Geometry check sheet. Reference: the model listing, model coordinates, mm. A direction names the side the tool comes from. Round coordinates to 2 decimals unless told otherwise and drop trailing zeros. Order: outer loops, then holes, each group sorted by start corner. A loop starts at its lowest first (then second) coordinate and runs counter-clockwise, first axis right, second up. Notation, with made-up numbers: (27.25, 81) - (74.25, 81) arc R38 ccw to (74.25, 119) - close; hole circle Ø1 at (25.25, -9). An arc over 180 degrees is marked (long way). Write each question's results on one line, items separated by ' | '.
```python
from build123d import *

# Parameters (mm, degrees)
SKETCH041_W     = 14
SKETCH041_H     = 48
PAD017_DEPTH    = 2
SKETCH043_W     = 10.7
SKETCH043_H     = 16.95
SKETCH043_H_2   = 5
PAD018_DEPTH    = 2
SKETCH044_W     = 10.7
SKETCH044_H     = 2
PAD019_DEPTH    = 11
SKETCH045_R     = 1.6
POCKET019_DEPTH = 5
CHAMFER002_SIZE = 1.5
FILLET006_R     = 1.5
FILLET007_R     = 1
FILLET008_R     = 1


with BuildPart() as part:
    # Sketch041 → Pad017 (new body)
    with BuildSketch(Plane.XY):
        with Locations((-17, -34)):
            Rectangle(SKETCH041_W, SKETCH041_H)
    extrude(amount=PAD017_DEPTH)

    # Sketch043 (on Face5 of Pad017) → Pad018 (join)
    with BuildSketch(Plane(origin=(0, 0, 0), x_dir=(1, 0, 0), z_dir=(0, 0, -1))):
        with Locations((-17, 26.525)):
            Rectangle(SKETCH043_W, SKETCH043_H)
        with Locations((-17, 53.45)):
            Rectangle(SKETCH043_W, SKETCH043_H_2)
    extrude(amount=PAD018_DEPTH)

    # Sketch044 (on Face4 of Pad018) → Pad019 (join)
    with BuildSketch(Plane(origin=(0, 0, 0), x_dir=(1, 0, 0), z_dir=(0, 0, -1))):
        with Locations((-17, 11)):
            Rectangle(SKETCH044_W, SKETCH044_H)
    extrude(amount=PAD019_DEPTH)

    # Sketch045 (on Face5 of Pad019) → Pocket019 (cut)
    with BuildSketch(Plane.XY.offset(2)):
        with Locations((-14.5, -30)):
            Circle(SKETCH045_R)
        with Locations((-17, -54.25)):
            Circle(SKETCH045_R)
    extrude(amount=-POCKET019_DEPTH, mode=Mode.SUBTRACT)

    # Chamfer002
    chamfer002_edges = [part.edges().sort_by_distance(p)[0] for p in [
        (-16.1, -30, 2),
        (-18.6, -54.25, 2),
    ]]
    chamfer(chamfer002_edges, length=CHAMFER002_SIZE)

    # Fillet006
    fillet006_edges = [part.edges().sort_by_distance(p)[0] for p in [
        (-10, -58, 1),
        (-24, -58, 1),
        (-24, -10, 1),
        (-10, -10, 1),
    ]]
    fillet(fillet006_edges, radius=FILLET006_R)

    # Fillet007
    fillet007_edges = [part.edges().sort_by_distance(p)[0] for p in [
        (-24, -34, 2),
    ]]
    fillet(fillet007_edges, radius=FILLET007_R)

    # Fillet008
    fillet008_edges = [part.edges().sort_by_distance(p)[0] for p in [
        (-22.35, -55.95, -1),
        (-11.65, -55.95, -1),
        (-22.35, -35, -1),
        (-11.65, -35, -1),
        (-11.65, -12, -5.5),
        (-22.35, -12, -5.5),
        (-11.65, -18.05, -1),
        (-22.35, -18.05, -1),
        (-22.35, -50.95, -1),
        (-11.65, -50.95, -1),
    ]]
    fillet(fillet008_edges, radius=FILLET008_R)


solid = part.part
```
(1) Section check B-B (y = -30). Record the cut outline in (x, z), then the cut area to 3 significant figures.
Answers follow:
outline: (-24, 0) - (-22.35, 0) - (-22.35, -2) - (-16.1, -2) - (-16.1, 0.5) - (-17.6, 2) - (-23, 2) arc R1 ccw to (-24, 1) - close; (-12.9, -2) - (-11.65, -2) - (-11.65, 0) - (-10, 0) - (-10, 1) arc R1 ccw to (-11, 2) - (-11.4, 2) - (-12.9, 0.5) - close | area: 33.9 mm²
(2) Material ranges on line 1 (Y direction, x = -14.5, z = -1.1); line 2 (Y direction, x = -20.75, z = -1.25); line 3 (Z direction, x = -18.5, y = -21), recorded low to high.
Answers follow:
line 1: -55.95 to -50.95, -35 to -31.6, -28.4 to -18.05, -12 to -10 | line 2: -55.95 to -50.95, -35 to -18.05, -12 to -10 | line 3: -2 to 2
(3) Section check C-C (y = -16.5). Record the cut outline in (x, z), then the cut area to 3 significant figures.
Answers follow:
outline: (-24, 0) - (-10, 0) - (-10, 1) arc R1 ccw to (-11, 2) - (-23, 2) arc R1 ccw to (-24, 1) - close | area: 27.6 mm²
(4) Section check A-A (z = -1.5). Record the cut outline in (x, y), then the cut area to 3 significant figures.
Answers follow:
outline: (-22.35, -54.95) arc R1 ccw to (-21.35, -55.95) - (-12.65, -55.95) arc R1 ccw to (-11.65, -54.95) - (-11.65, -51.95) arc R1 ccw to (-12.65, -50.95) - (-21.35, -50.95) arc R1 ccw to (-22.35, -51.95) - close; (-22.35, -34) arc R1 ccw to (-21.35, -35) - (-12.65, -35) arc R1 ccw to (-11.65, -34) - (-11.65, -19.05) arc R1 ccw to (-12.65, -18.05) - (-21.35, -18.05) arc R1 ccw to (-22.35, -19.05) - close; (-22.35, -11) arc R1 ccw to (-21.35, -12) - (-12.65, -12) arc R1 ccw to (-11.65, -11) - (-11.65, -10) - (-22.35, -10) - close; hole circle Ø3.2 at (-17, -54.25); hole circle Ø3.2 at (-14.5, -30) | area: 238 mm²
(5) Depth check by flat-ended pin: pin 1 Ø0.8 at (y, z) = (-10.5, -7.5) entering from +X; pin 2 Ø0.6 at (x, z) = (-18, -1) entering from -Y; pin 3 Ø2 at (x, y) = (-13, -31) entering from -Z. Enter the tip coordinate at first touch or a pass-through.
Answers follow:
pin 1: x = -11.65 | pin 2: y = -55.95 | pin 3: z = -2
(6) Section check D-D (z = -9). Record the cut outline in (x, y), then the cut area to 3 significant figures.
Answers follow:
outline: (-22.35, -11) arc R1 ccw to (-21.35, -12) - (-12.65, -12) arc R1 ccw to (-11.65, -11) - (-11.65, -10) - (-22.35, -10) - close | area: 21.0 mm²
(7) Draft check along Y on faces 4 (the face through (-16.923, -10.301, 1.715)), 5 (the face through (-17, -39, 0)), 6 (the face through (-11.65, -26, -1)). Enter one of: released by +Y, released by -Y, zero draft, split by the parting line, or undercut.
Answers follow:
face 4: released by +Y | face 5: undercut | face 6: zero draft
(8) Access from +Z, -Z, +X, -X, +Y, -Y to the whole of each face (thin tool, end or side, straight path). Record for faces 1 (the face through (-11.951, -34.715, -1.014)), 2 (the face through (-22.065, -11.699, -5.577)), 3 (the face through (-11.65, -10.5, -5.4)).
Answers follow:
face 1: -Z, +X | face 2: -Z, -X | face 3: -Z, +X, +Y, -Y
